Autodesk Inventor part; units mm, degrees
ref_plane "Work Plane2" through (0, -410, -108) normal (0, 0, -1) x (0, 1, 0)
ref_plane "Work Plane3" through (0, -410, 1041.034) normal (0, 0, 1) x (1, 0, 0)
ref_plane "Work Plane4" through (29, 140, 933.034) normal (1, 0, 0) x (0, 1, 0)
ref_plane "Work Plane1" through (0, 0, 0) normal (0, 0, 1) x (1, 0, 0)
sketch "Sketch1" plane through (0, 0, 0) normal (0, 0, 1) x (1, 0, 0)
  line L0 (29, 140) -> (29, 248)
  line L1 (29, 248) -> (58, 248)
  line L2 (29, 248) -> (58, 248)
  line L3 (58, 248) -> (58, 410)
  line L4 (0, 410) -> (58, 410)
  line L5 (0, -410) -> (0, 410)
  line L6 (58, -410) -> (0, -410)
  line L7 (58, -410) -> (58, -252)
  line L8 (58, -252) -> (29, -252)
  line L9 (29, -252) -> (29, -144)
  line L10 (29, -144) -> (58, -144)
  line L11 (58, -144) -> (58, 140)
  line L12 (58, 140) -> (29, 140)
  line L13 (29, 140) -> (29, 248)
  line L14 (58, 140) -> (29, 140)
  line L15 (58, 140) -> (0, 140)
  line L16 (0, 140) -> (0, 248)
  line L17 (0, 248) -> (58, 248)
  line L18 (58, 248) -> (58, 140)
  point P0 (0, 0)
ref_plane "Work Plane2" through (0, -410, -108) normal (0, 0, -1) x (0, 1, 0)
ref_plane "Work Plane3" through (0, -410, 1041.034) normal (0, 0, 1) x (1, 0, 0)
extrude "Extrusion1" add sketch "Sketch1" along normal up to surface (1149.034 mm away) from surface at -108 contours L15 L5 L17 L0 | L0 L1 L18 L12
sketch "Sketch2" plane through (0, 140, 1041.034) normal (-1, 0, 0) x (0, 0, 1)
  line L0 (-1041.034, -550) -> (-1041.034, 270)
  line L1 (-1149.034, 270) -> (-1041.034, 270)
  line L2 (-1149.034, -550) -> (-1149.034, 270)
  line L3 (-1041.034, -550) -> (-1149.034, -550)
  line L4 (-333.034, -550) -> (-333.034, 270)
  line L5 (-441.034, 270) -> (-333.034, 270)
  line L6 (-441.034, -550) -> (-441.034, 270)
  line L7 (-333.034, -550) -> (-441.034, -550)
  line L8 (0, -550) -> (0, 270)
  line L9 (-108, 270) -> (0, 270)
  line L10 (-108, -550) -> (-108, 270)
  line L11 (0, -550) -> (-108, -550)
  line L12 (0, 0) -> (0, 108)
  line L13 (-1149.034, 108) -> (0, 108)
  line L14 (-1149.034, 108) -> (-1149.034, 0)
  line L15 (-1149.034, 0) -> (0, 0)
  line L16 (-1041.034, 0) -> (-1149.034, 0)
  line L17 (-1149.034, 0) -> (-1149.034, 108)
  line L18 (-1149.034, 108) -> (-1041.034, 108)
  line L19 (-1041.034, 108) -> (-1041.034, 0)
  line L20 (-1149.034, 108) -> (0, 108)
  line L21 (-441.034, 108) -> (-333.034, 108)
  line L22 (-333.034, 108) -> (-333.034, 0)
  line L23 (-333.034, 0) -> (-441.034, 0)
  line L24 (-441.034, 0) -> (-441.034, 108)
  line L25 (-1149.034, 0) -> (0, 0)
  line L26 (0, 0) -> (0, 108)
  line L27 (-108, 0) -> (0, 0)
  line L28 (0, 0) -> (0, 108)
  line L29 (0, 108) -> (-108, 108)
  line L30 (-108, 108) -> (-108, 0)
  point P0 (-1041.034, -140)
ref_plane "Work Plane4" through (29, 140, 933.034) normal (1, 0, 0) x (0, 1, 0)
extrude "Extrusion2" cut sketch "Sketch2" against normal up to surface (29 mm away) contours L15 L2 L13 L0 | L6 L13 L4 L15 | L10 L13 L8 L15
properties part number "horizontalUnderSink" material "Wood (Birch)"
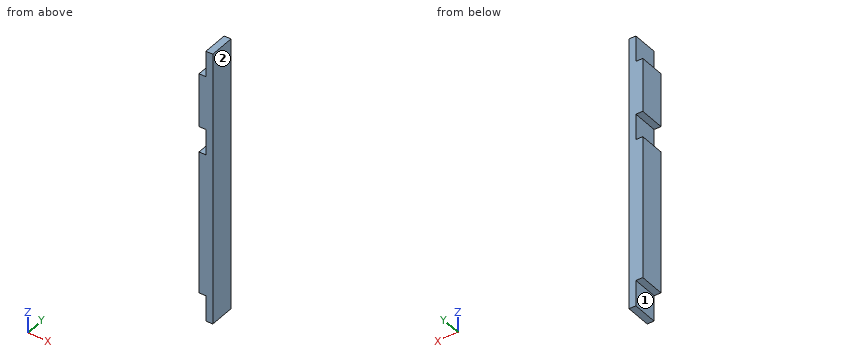
Here's how the part is built. I have some questions about the finished solid (model axes, mm). Face numbers are marked on the shaded views. A direction names the side the tool comes from. Coordinates: 2 decimals unless noted, no trailing zeros. Order: outer loops, then holes, each group sorted by start corner. A loop starts at its lowest first (then second) coordinate and runs counter-clockwise, first axis right, second up. Notation, with made-up numbers: (83.25, -25) - (132.25, -25) arc R21 cw to (132.25, -11) - close; hole circle Ø6 at (-13, 28.25). An arc over 180 degrees is marked (long way). Use CSV: the item, a comma, the result in double quotes. Start each with the question number.
1. Suppose I cut it at B-B on y = 235.5. List the corners of the cut face in (x, z) for me.
2. Please list where these lines run through material, in increasing order: line 1 (Z direction, x = 28.5, y = 181.5); line 2 (X direction, y = 232.5, z = 630). Write a range as from..to.
3. Suppose I cut it at C-C on z = -25.5. List the corners of the cut face in (x, y) for me, then the cut area to 3 significant figures.
4. For the marked faces 1 and 2, which set-ups out of +Z, -Z, +X, -X, +Y, -Y let a thin tool reach every point of the face, with its end or its side?
5. I'm going to push flat-ended pins straight in: pin 1 (8.5 mm diameter, centred on x = 14.5, y = 184, fed in from +Z); pin 2 (8.5 mm diameter, centred on x = 14.5, y = 169.5, fed in from -Z). Where does each tip first touch, or does it pass through?
6. Suppose I cut it at A-A on x = 17. List the corners of the cut face in (y, z) for me.
Output:
1,outline,"(0, 0) - (29, 0) - (29, -108) - (58, -108) - (58, 1041.03) - (29, 1041.03) - (29, 933.03) - (0, 933.03) - (0, 708) - (29, 708) - (29, 600) - (0, 600) - close"
2,line 1,"z = 0..600, 708..933.03"
2,line 2,"x = 29..58"
3,outline,"(29, 140) - (58, 140) - (58, 248) - (29, 248) - close"
3,area,"3,130 mm2"
4,face 1,"-Z, -X, +Y, -Y"
4,face 2,"+Z, -Z, +X, +Y, -Y"
5,pin 1,"stops at z = 933.03"
5,pin 2,"stops at z = 0"
6,outline,"(140, 0) - (248, 0) - (248, 600) - (140, 600) - close; (140, 708) - (248, 708) - (248, 933.03) - (140, 933.03) - close"
